For this review, take the finished solid that the model builds, in its own axes (mm). Face numbers are marked on the shaded views. Round coordinates to 2 decimals unless told otherwise and drop trailing zeros. Order: outer loops, then holes, each group sorted by start corner. A loop starts at its lowest first (then second) coordinate and runs counter-clockwise, first axis right, second up. Notation, with made-up numbers: (-24.5, 33.25) - (-7.5, 33.25) arc R14 ccw to (-7.5, 51.25) - close; hole circle Ø3 at (-32, 1). An arc over 180 degrees is marked (long way). One line per question, with ' | ' between items.
```python
from build123d import *

# Parameters (mm, degrees)
F0_R     = 45
F0_R_2   = 40
F1_DEPTH = 2
F0_R_3   = 10
F0_R_4   = 5
F0_R_5   = 1.7
F0_R_6   = 4.4
F0_R_7   = 2.9
F2_DEPTH = 2


with BuildPart() as f1:
    # F0 (on Top) → F1 (new body, symmetric)
    with BuildSketch(Plane.XY):
        Circle(F0_R)
        Circle(F0_R_2, mode=Mode.SUBTRACT)
    extrude(amount=F1_DEPTH, both=True)

    # F0 (on Top) → F2 (join, through all)
    with BuildSketch(Plane.XY):
        Circle(F0_R_2)
        with Locations((-17.07316, -17.07316)):
            Circle(F0_R_3, mode=Mode.SUBTRACT)
        with Locations((0, -24.145094)):
            Circle(F0_R_4, mode=Mode.SUBTRACT)
        with Locations((17.07316, -17.07316)):
            Circle(F0_R_3, mode=Mode.SUBTRACT)
        with Locations((0, -9.8)):
            Circle(F0_R_5, mode=Mode.SUBTRACT)
        with Locations((-24.145094, 0)):
            Circle(F0_R_4, mode=Mode.SUBTRACT)
        with Locations((-9.8, 0)):
            Circle(F0_R_5, mode=Mode.SUBTRACT)
        with Locations((-17.07316, 17.07316)):
            Circle(F0_R_3, mode=Mode.SUBTRACT)
        Circle(F0_R_6, mode=Mode.SUBTRACT)
        with Locations((9.8, 0)):
            Circle(F0_R_5, mode=Mode.SUBTRACT)
        with Locations((0, 9.8)):
            Circle(F0_R_5, mode=Mode.SUBTRACT)
        with Locations((17.07316, 17.07316)):
            Circle(F0_R_3, mode=Mode.SUBTRACT)
        with Locations((24.145094, 0)):
            Circle(F0_R_4, mode=Mode.SUBTRACT)
        with Locations((0, 24.145094)):
            Circle(F0_R_4, mode=Mode.SUBTRACT)
        Circle(F0_R_6)
        Circle(F0_R_7, mode=Mode.SUBTRACT)
    extrude(amount=-F2_DEPTH)


solid = f1.part
```
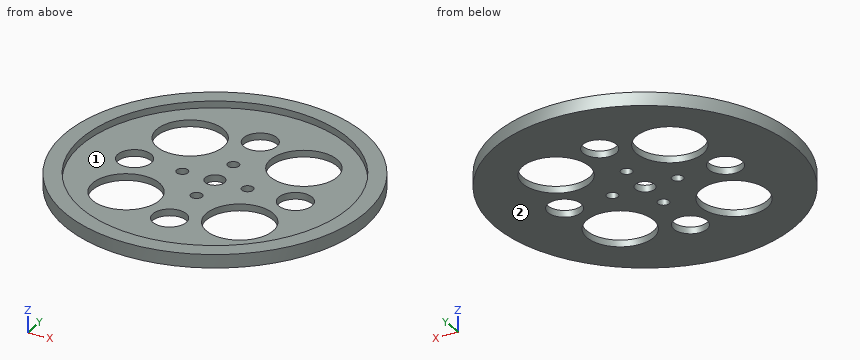
(1) We need section A-A on x = 9.8. State the section outline as (y, z) points.
Output values:
outline: (-43.92, -2) - (-23.94, -2) - (-23.94, 0) - (-38.78, 0) - (-38.78, 2) - (-43.92, 2) - close; (-10.21, -2) - (-1.7, -2) - (-1.7, 0) - (-10.21, 0) - close; (1.7, -2) - (10.21, -2) - (10.21, 0) - (1.7, 0) - close; (23.94, -2) - (43.92, -2) - (43.92, 2) - (38.78, 2) - (38.78, 0) - (23.94, 0) - close
(2) Mouldability with a two-part tool opening along Y and no side actions: class the marked faces 1 and 2 as released by +Y, released by -Y, zero draft, split by the parting line, or undercut.
Output values:
face 1: undercut | face 2: zero draft
(3) We need section D-D on x = 0. State the section outline as (y, z) points, plus the area to 3 significant figures.
Output values:
outline: (-45, -2) - (-29.15, -2) - (-29.15, 0) - (-40, 0) - (-40, 2) - (-45, 2) - close; (-19.15, -2) - (-11.5, -2) - (-11.5, 0) - (-19.15, 0) - close; (-8.1, -2) - (-2.9, -2) - (-2.9, 0) - (-8.1, 0) - close; (2.9, -2) - (8.1, -2) - (8.1, 0) - (2.9, 0) - close; (11.5, -2) - (19.15, -2) - (19.15, 0) - (11.5, 0) - close; (29.15, -2) - (45, -2) - (45, 2) - (40, 2) - (40, 0) - (29.15, 0) - close | area: 135 mm^2
(4) Insertion check: pin 1 (18 mm diameter, centred on x = -17.07, y = 17.07, fed in from +Z); pin 2 (9.5 mm diameter, centred on x = 0, y = 0, fed in from -Z); pin 3 (23 mm diameter, centred on x = 17.07, y = 17.07, fed in from +Z). Each pin has a flat end and moves straight along its axis. Give the tip position at first contact, or say it passes through.
Output values:
pin 1: through | pin 2: z = -2 | pin 3: z = 0
(5) We need section C-C on z = -0.9. Give the number of separate pieces and of enclosed holes in the cut face, plus the area to 3 significant figures.
Output values:
separate pieces: 1 | enclosed holes: 13 | area: 4,730 mm^2
(6) For probe 1 along Y at (x, z) = (0, -0.35); probe 2 along X at (y, z) = (-15, -1.05); probe 3 along Y at (x, z) = (12, -0.85), list the stretches that pass through material, from the lowest coordinate up. Write a range as [from, to].
Output values:
probe 1: [-45, -29.15], [-19.15, -11.5], [-8.1, -2.9], [2.9, 8.1], [11.5, 19.15], [29.15, 45] | probe 2: [-42.43, -26.86], [-7.29, 7.29], [26.86, 42.43] | probe 3: [-43.37, -25.69], [-8.46, 8.46], [25.69, 43.37]
